Could you check a few things on this model? Use its own coordinates, in mm. Round coordinates to 2 decimals unless told otherwise and drop trailing zeros. Return JSON: item names as keys, results as strings.
from build123d import *

# Parameters (mm, degrees)
F0_R     = 3
F0_R_2   = 2.5
F1_DEPTH = 655
F2_R     = 2
F3_R     = 7


# Not quite as in the source:
# - a feature names something its author has since deleted; it is built from what else it names


with BuildPart() as f1:
    # F0 (on Top) → F1 (new body)
    with BuildSketch(Plane.XY):
        with BuildLine():
            Line((18.15, -15), (30, -15))
            Line((30, -15), (30, -3.15))
            Line((30, -3.15), (27.5, -3.15))
            Line((27.5, -3.15), (27.5, -5.15))
            Line((27.5, -5.15), (21.5477069044, -5.15))
            ThreePointArc((21.5477069044, -5.15), (19.5, 0), (21.5477069044, 5.15))
            Line((21.5477069044, 5.15), (27.5, 5.15))
            Line((27.5, 5.15), (27.5, 3.15))
            Line((27.5, 3.15), (30, 3.15))
            Line((30, 3.15), (30, 15))
            Line((30, 15), (18.15, 15))
            Line((18.15, 15), (18.15, 12.5))
            Line((18.15, 12.5), (20.15, 12.5))
            Line((20.15, 12.5), (20.15, 6.5477069044))
            ThreePointArc((20.15, 6.5477069044), (15, 4.5), (9.85, 6.5477069044))
            Line((9.85, 6.5477069044), (9.85, 12.5))
            Line((9.85, 12.5), (11.85, 12.5))
            Line((11.85, 12.5), (11.85, 15))
            Line((11.85, 15), (-11.85, 15))
            Line((-11.85, 15), (-11.85, 12.5))
            Line((-11.85, 12.5), (-9.85, 12.5))
            Line((-9.85, 12.5), (-9.85, 6.5477069044))
            ThreePointArc((-9.85, 6.5477069044), (-15, 4.5), (-20.15, 6.5477069044))
            Line((-20.15, 6.5477069044), (-20.15, 12.5))
            Line((-20.15, 12.5), (-18.15, 12.5))
            Line((-18.15, 12.5), (-18.15, 15))
            Line((-18.15, 15), (-30, 15))
            Line((-30, 15), (-30, 3.15))
            Line((-30, 3.15), (-27.5, 3.15))
            Line((-27.5, 3.15), (-27.5, 5.15))
            Line((-27.5, 5.15), (-21.5477069044, 5.15))
            ThreePointArc((-21.5477069044, 5.15), (-19.5, 0), (-21.5477069044, -5.15))
            Line((-21.5477069044, -5.15), (-27.5, -5.15))
            Line((-27.5, -5.15), (-27.5, -3.15))
            Line((-27.5, -3.15), (-30, -3.15))
            Line((-30, -3.15), (-30, -15))
            Line((-30, -15), (-18.15, -15))
            Line((-18.15, -15), (-18.15, -12.5))
            Line((-18.15, -12.5), (-20.15, -12.5))
            Line((-20.15, -12.5), (-20.15, -6.5477069044))
            ThreePointArc((-20.15, -6.5477069044), (-15, -4.5), (-9.85, -6.5477069044))
            Line((-9.85, -6.5477069044), (-9.85, -12.5))
            Line((-9.85, -12.5), (-11.85, -12.5))
            Line((-11.85, -12.5), (-11.85, -15))
            Line((-11.85, -15), (11.85, -15))
            Line((11.85, -15), (11.85, -12.5))
            Line((11.85, -12.5), (9.85, -12.5))
            Line((9.85, -12.5), (9.85, -6.5477069044))
            ThreePointArc((9.85, -6.5477069044), (15, -4.5), (20.15, -6.5477069044))
            Line((20.15, -6.5477069044), (20.15, -12.5))
            Line((20.15, -12.5), (18.15, -12.5))
            Line((18.15, -12.5), (18.15, -15))
        make_face()
        with Locations((-25, -10)):
            Circle(F0_R, mode=Mode.SUBTRACT)
        with Locations((25, -10)):
            Circle(F0_R, mode=Mode.SUBTRACT)
        with Locations((-15, 0)):
            Circle(F0_R_2, mode=Mode.SUBTRACT)
        with Locations((-25, 10)):
            Circle(F0_R, mode=Mode.SUBTRACT)
        Polygon((-7, 7), (-7, 12.5), (0, 12.5), (7, 12.5), (7, 7), (10, 0), (7, -7), (7, -12.5), (0, -12.5), (-7, -12.5), (-7, -7), (-10, 0), align=None, mode=Mode.SUBTRACT)
        with Locations((15, 0)):
            Circle(F0_R_2, mode=Mode.SUBTRACT)
        with Locations((25, 10)):
            Circle(F0_R, mode=Mode.SUBTRACT)
    extrude(amount=F1_DEPTH)

    # F2
    f2_edges = [f1.edges().sort_by_distance(p)[0] for p in [
        (-7, 12.5, 327.5),
        (7, 12.5, 327.5),
    ]]
    fillet(f2_edges, radius=F2_R)

    # F3
    f3_edges = [f1.edges().sort_by_distance(p)[0] for p in [
        (-7, 7, 327.5),
        (-10, 0, 327.5),
        (7, 7, 327.5),
        (10, 0, 327.5),
    ]]
    fillet(f3_edges, radius=F3_R)


solid = f1.part
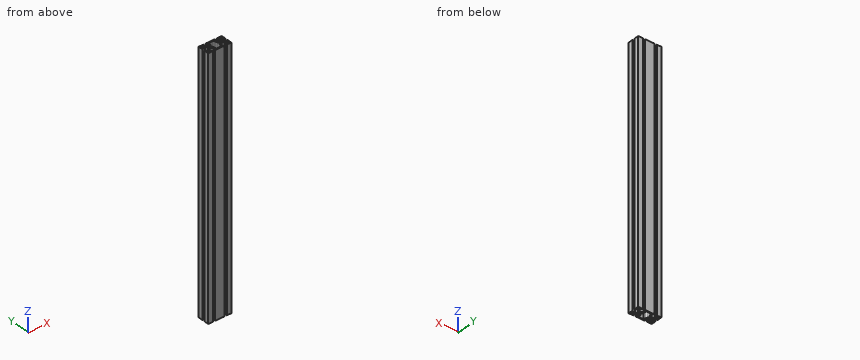
1) If I drill on probe 1 along Y at (x, z) = (-25, 363.5); probe 2 along X at (y, z) = (9.5, 466); probe 3 along Y at (x, z) = (2, 73), over which ranges is the centre line in solid material (lowest first)? Write a range as [from, to].
Return value:
{"probe 1": "[-15, -13], [-7, -5.15], [5.15, 7], [13, 15]", "probe 2": "[-30, -27.96], [-22.04, -20.15], [-9.85, -7], [7, 9.85], [20.15, 22.04], [27.96, 30]", "probe 3": "[-15, -12.5], [12.5, 15]"}
2) Will this pin go through, and if not, where does the flat tip stop? pin 1 Ø2 at (y, z) = (1.5, 76.5) entering from -X.
Return value:
{"pin 1": "x = -19.93"}
3) I want a section at A-A, the plane z = 230.5. Count the separate pieces of the cut face and the enclosed holes in it, and give its area (3 significant figures).
Return value:
{"separate pieces": "1", "enclosed holes": "7", "area": "710 mm²"}
